Could you check a few things on this model? Use its own coordinates, in mm. Face numbers are marked on the shaded views. A direction names the side the tool comes from. Give positions to 0.01 mm unless a question says otherwise; leave off trailing zeros. Loops run counter-clockwise (first coordinate to the right, second up) from the corner with the lowest first, then second, coordinate; pieces in that order, holes last. Notation, with made-up numbers: M -11.5,75.25 L 41.5,75.25 A28 cw 41.5,104.25 Z; hole C -19.5,-32 d6. An arc over 180 degrees is marked long. Write each question's results on one line, items separated by ' | '. Start each with the question number.
from build123d import *

# Parameters (mm, degrees)
F2_R     = 20
F3_DEPTH = 6
F4_T     = 1
F5_R     = 2
F7_D     = 4.5


# Not quite as in the source:
# - a shell that OpenCascade refuses in one call is made with other operations: the cavity is built on its own and cut out


with BuildPart() as f1:
    # F0 (on Front) → F1 (revolve)
    with BuildSketch(Plane.XZ):
        Polygon((0, 12.5), (0, 0), (73.4, 0), (73.4, 29.5), (67.7, 29.5), (67.7, 44), (66.5, 44), (66.5, 29), (18.5, 29), (6.5, 12.5), align=None)
    revolve(axis=Axis((36.7, 0, 0), (-1, 0, 0)))

    # F2 (on face) → F3 (cut)
    with BuildSketch(Plane.YZ.offset(73.4)):
        Circle(F2_R)
    extrude(amount=-F3_DEPTH, mode=Mode.SUBTRACT)

    # F4: shell of thickness 1, made by hand


with BuildPart() as f4_core1:
    # F4_t2: copy of F1
    add(f1.part)

    # the walls: a layer under each face that stays
    f4_faces = [f4_core1.faces().sort_by_distance(p)[0] for p in [
        (3.25, 0, -12.5),
        (12.5, 0, -20.75),
        (42.5, 0, -29),
        (66.5, -29.3333333333, -29.3333333333),
        (67.1, 0, -44),
        (67.7, -29.3333333333, 29.3333333333),
        (70.55, 0, -29.5),
        (73.4, -19.6666666667, 19.6666666667),
        (70.4, -20, 0),
    ]]
    thicken(f4_faces, amount=-F4_T, mode=Mode.SUBTRACT)

    # F4_s3 → F4_t4 (revolve, cut)
    with BuildSketch(Plane.XZ):
        Polygon((6.4919126392, 12.515881717), (6.5, 11.5), (7.0092245917, 11.5), (7.3087360843, 11.9118283023), align=None)
    revolve(axis=Axis((6.5, 0, 0), (-1, 0, 0)), mode=Mode.SUBTRACT)

    # F4_s5 → F4_t6 (revolve, cut)
    with BuildSketch(Plane.XZ):
        Polygon((66.49, 29.01), (66.5, 28), (67.5, 28), (67.5, 29), align=None)
    revolve(axis=Axis((66.5, 0, 0), (-1, 0, 0)), mode=Mode.SUBTRACT)

    # F4_s7 → F4_t8 (revolve, cut)
    with BuildSketch(Plane.XZ):
        Polygon((67.71, 29.51), (66.7, 29.5), (66.7, 28.5), (67.7, 28.5), align=None)
    revolve(axis=Axis((67.7, 0, 0), (-1, 0, 0)), mode=Mode.SUBTRACT)


with BuildPart() as f1_1:
    add(f1.part)

    # what is left inside the walls is the cavity
    f4_cavity = [f4_core1.part.solids().sort_by_distance(p)[0] for p in [
        (50.669742, 0, -27.99),
    ]]
    add(f4_cavity, mode=Mode.SUBTRACT)

    # F5
    f5_edges = [f1_1.edges().sort_by_distance(p)[0] for p in [
        (73.4, 0, -29.5),
        (73.4, -20, 0),
    ]]
    fillet(f5_edges, radius=F5_R)

    # F7 (through all)
    with Locations(Plane.YZ.offset(67.7)):
        with Locations((0, 39), (0, -39)):
            Hole(F7_D / 2)


solid = f1_1.part
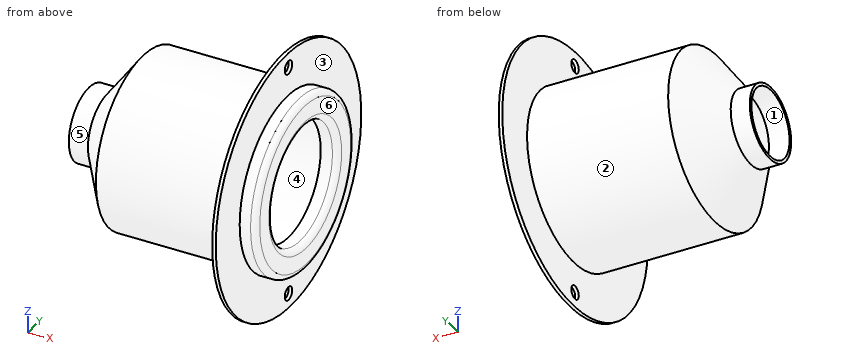
1) I'm going to push flat-ended pins straight in: P1, Ø8, axis at x = 63, z = -24, coming from the +Y side; P2, Ø3, axis at x = 53.5, y = -3.5, coming from the -Z side; P3, Ø3, axis at x = 42.5, z = 18, coming from the -Y side. Where does each tip first touch, or does it pass through?
2) If we section it at A-A on z = -39: Write out the boundary of the cut face in (x, y), plus the area to 3 significant figures.
3) Please list where these lines run through material, in increasing order: line 1 (X direction, y = -14, z = -26); line 2 (X direction, y = 15.5, z = -21.5); line 3 (X direction, y = 6.5, z = -23). Write a range as from..to.
4) Which directions (+Z, -Z, +X, -X, +Y, -Y) give clear straight access to the entire face, cutting with the end or side of a thin tool? Please do the marked faces 4, 5 and 6.
5) If we section it at B-B on x = 34: Write out the boundary of the cut face in (y, z), plus the area to 3 significant figures.
6) If we section it at C-C on y = -36.5: Write out the boundary of the cut face in (x, z), plus the area to 3 significant figures.
7) Thinking about a two-plate mould opening in Y: for the marked faces 1, 2 and 3, which applies, pulls with the +Y half, pulls with the -Y half, needs draft (parallel to the pull), parting line crosses it, or undercut?
Calculated:
1) P1: stops at y = 38.07 | P2: stops at z = -28.93 | P3: stops at y = -23.85
2) outline: M 66.5,-20.37 L 67.7,-20.37 L 67.7,-2.25 L 66.5,-2.25 Z; M 66.5,2.25 L 67.7,2.25 L 67.7,20.37 L 66.5,20.37 Z | area: 43.5 mm2
3) line 1: x = 66.5..67.7 | line 2: x = 16.69..17.92, 72.4..73.4 | line 3: x = 14.79..16.03, 72.4..73.4
4) face 4: none | face 5: -X | face 6: +Z, -Z, +X, +Y, -Y
5) outline: C 0,0 d58; hole C 0,0 d56 | area: 179 mm2
6) outline: M 66.5,-24.57 L 67.7,-24.57 L 67.7,24.57 L 66.5,24.57 Z | area: 59.0 mm2
7) face 1: undercut | face 2: parting line crosses it | face 3: needs draft
